Design review of the part built by this model. Coordinates are the model's own, in mm. Face numbers are marked on the shaded views. A direction names the side the tool comes from. Give positions to 0.01 mm unless a question says otherwise; leave off trailing zeros. Loops run counter-clockwise (first coordinate to the right, second up) from the corner with the lowest first, then second, coordinate; pieces in that order, holes last. Notation, with made-up numbers: M 70.25,-26.75 L 92.25,-26.75 A22 cw 92.25,-15.75 Z; hole C 39,-21 d6. An arc over 180 degrees is marked long. Use a Markdown table: item, result. Add a question column.
(1) Add section A-A, the plane y = 13.25. Give the boundary of the cut face in (x, z), then the cut area to 3 significant figures.
(2) Add section B-B, the plane x = 27. Give the boundary of the cut face in (y, z), then the cut area to 3 significant figures.
(3) Insertion check: pin 1 Ø1.2 at (x, z) = (29, 2) entering from +Y; pin 2 Ø8 at (x, y) = (38.5, 9.5) entering from +Z; pin 3 Ø0.8 at (y, z) = (16, 3) entering from +X. Each pin has a flat end and moves straight along its axis. Give the tip position at first contact, or say it passes through.
(4) For the marked faces 1, 2 and 3, list the 3-axis set-ups (+Z, -Z, +X, -X, +Y, -Y) from which the entire face can be reached by the end or side of a thin tool; tool diameter is ignored.
(5) Draft analysis for pull direction X (two halves, no side actions). For the marked faces 4 and 5, state which applies: pulls with the +X half, pulls with the -X half, needs draft (parallel to the pull), parting line crosses it, or undercut.
(6) For probe 1 along X at (y, z) = (8.5, 1.7); probe 2 along X at (y, z) = (10.5, 3.2); probe 3 along Y at (x, z) = (31.5, 3.8), list the stretches that pass through material, from the lowest coordinate up.
```python
from build123d import *

# Parameters (mm, degrees)
SKETCH1_W           = 43
SKETCH1_H           = 18
BOSS_EXTRUDE1_DEPTH = 4.5
SKETCH2_W           = 22
SKETCH2_H           = 3
CUT_EXTRUDE1_DEPTH  = 47.832147079
SKETCH3_W           = 22
SKETCH3_H           = 3
CUT_EXTRUDE2_DEPTH  = 47.832147079
CUT_EXTRUDE3_DEPTH  = 3.5
CUT_EXTRUDE4_DEPTH  = 47.832147079
SKETCH6_W           = 1.5
SKETCH6_H           = 10
CUT_EXTRUDE5_DEPTH  = 17
CHAMFER1_SIZE       = 0.4
CHAMFER2_SIZE       = 0.4


with BuildPart() as part:
    # Sketch1 → Boss-Extrude1 (new body)
    with BuildSketch(Plane(origin=(0, 0, 0), x_dir=(-1, 0, 0), z_dir=(0, 0, -1))):
        with Locations((-21.5, 9)):
            Rectangle(SKETCH1_W, SKETCH1_H)
    extrude(amount=-BOSS_EXTRUDE1_DEPTH)

    # Sketch2 → Cut-Extrude1 (cut, through all)
    with BuildSketch(Plane.XY.offset(4.5)):
        with Locations((32, 1.5)):
            Rectangle(SKETCH2_W, SKETCH2_H)
    extrude(amount=-CUT_EXTRUDE1_DEPTH, mode=Mode.SUBTRACT)

    # Sketch3 → Cut-Extrude2 (cut, through all)
    with BuildSketch(Plane.XY.offset(4.5)):
        with Locations((32, 16.5)):
            Rectangle(SKETCH3_W, SKETCH3_H)
    extrude(amount=-CUT_EXTRUDE2_DEPTH, mode=Mode.SUBTRACT)

    # Sketch4 → Cut-Extrude3 (cut)
    with BuildSketch(Plane.XY.offset(4.5)):
        with BuildLine():
            Line((9.5, 14.8), (9.5, 7.3))
            ThreePointArc((9.5, 7.3), (7.5, 5.3), (5.5, 7.3))
            Line((5.5, 7.3), (5.5, 14.8))
            ThreePointArc((5.5, 14.8), (7.5, 16.8), (9.5, 14.8))
        make_face()
    extrude(amount=-CUT_EXTRUDE3_DEPTH, mode=Mode.SUBTRACT)

    # Sketch5 → Cut-Extrude4 (cut, through all)
    with BuildSketch(Plane(origin=(0, 0, 0), x_dir=(-1, 0, 0), z_dir=(0, 0, -1))):
        with BuildLine():
            Line((-6.300000004, 14.79990089), (-6.300621502, 7.27497794))
            ThreePointArc((-6.300621502, 7.27497794), (-7.500720608, 6.075077054), (-8.700621494, 7.27517616))
            Line((-8.700621494, 7.27517616), (-8.699999996, 14.80009911))
            ThreePointArc((-8.699999996, 14.80009911), (-7.49990089, 15.999999996), (-6.300000004, 14.79990089))
        make_face()
    extrude(amount=-CUT_EXTRUDE4_DEPTH, mode=Mode.SUBTRACT)

    # Sketch6 → Cut-Extrude5 (cut)
    with BuildSketch(Plane(origin=(43, 0, 0), x_dir=(0, 0, -1), z_dir=(1, 0, 0))):
        with Locations((-3.75, 9)):
            Rectangle(SKETCH6_W, SKETCH6_H)
    extrude(amount=-CUT_EXTRUDE5_DEPTH, mode=Mode.SUBTRACT)

    # Chamfer1
    chamfer1_edges = [part.edges().sort_by_distance(p)[0] for p in [
        (10.5, 0, 0),
        (21, 1.5, 0),
        (32, 3, 0),
        (43, 9, 0),
        (21, 16.5, 0),
        (32, 15, 0),
        (0, 9, 0),
        (10.5, 18, 0),
        (7.49990089, 15.999999996, 0),
        (8.700310745, 11.037637635, 0),
        (7.500720608, 6.075077054, 0),
        (6.300310753, 11.037439415, 0),
    ]]
    chamfer(chamfer1_edges, length=CHAMFER1_SIZE)

    # Chamfer2
    chamfer2_edges = [part.edges().sort_by_distance(p)[0] for p in [
        (21, 18, 2.45),
        (21, 0, 2.45),
        (0, 18, 2.45),
        (0, 0, 2.45),
    ]]
    chamfer(chamfer2_edges, length=CHAMFER2_SIZE)


solid = part.part
```
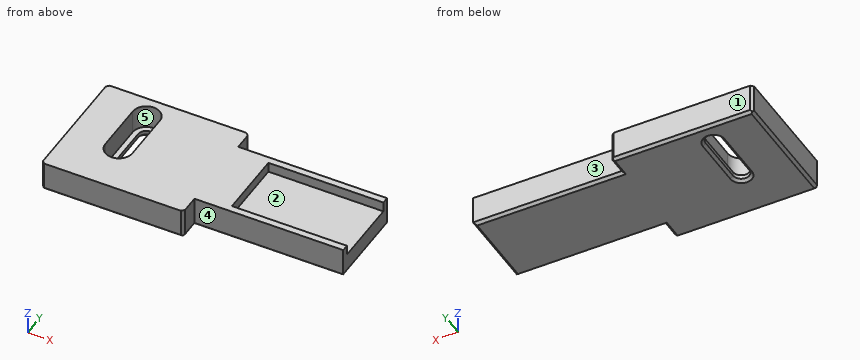
Established:
| question | item | result |
|---|---|---|
| 1 | outline | M 0,0.4 L 0.4,0 L 5.9,0 L 6.3,0.4 L 6.3,1 L 5.5,1 L 5.5,4.5 L 0,4.5 Z; M 8.7,0.4 L 9.1,0 L 42.6,0 L 43,0.4 L 43,3 L 26,3 L 26,4.5 L 9.5,4.5 L 9.5,1 L 8.7,1 Z |
| 1 | area | 151 mm^2 |
| 2 | outline | M 3,0.4 L 3.4,0 L 14.6,0 L 15,0.4 L 15,4.5 L 14,4.5 L 14,3 L 4,3 L 4,4.5 L 3,4.5 Z |
| 2 | area | 38.8 mm^2 |
| 3 | pin 1 | y = 15 |
| 3 | pin 2 | z = 3 |
| 3 | pin 3 | x = 21 |
| 4 | face 1 | +Z, -Z, +X, -X, +Y |
| 4 | face 2 | +Z, +X |
| 4 | face 3 | +Z, -Z, +X, +Y |
| 5 | face 4 | needs draft |
| 5 | face 5 | undercut |
| 6 | probe 1 | 0 to 5.5, 9.5 to 43 |
| 6 | probe 2 | 0 to 5.5, 9.5 to 26 |
| 6 | probe 3 | 3 to 4, 14 to 15 |
